```python
from build123d import *

# Parameters (mm, degrees)
BOSS_EXTRUDE1_DEPTH = 25.4
CUT_EXTRUDE1_REACH  = 3.587
SKETCH2_R           = 9.525
FILLET1_R           = 6.35
CUT_EXTRUDE2_REACH  = 33.75
SKETCH3_R           = 2.667


with BuildPart() as part:
    # Sketch1 → Boss-Extrude1 (new body)
    with BuildSketch(Plane(origin=(0, 0, 0), x_dir=(0, 0, -1), z_dir=(1, 0, 0))):
        Polygon((1.5875, 1.5875), (25.4, 1.5875), (25.4, 0), (0, 0), (0, 31.75), (1.5875, 31.75), align=None)
    extrude(amount=BOSS_EXTRUDE1_DEPTH)

    # Sketch2 → Cut-Extrude1 (cut, up to next)
    with BuildSketch(Plane(origin=(0, 0, -1.5875), x_dir=(-1, 0, 0), z_dir=(0, 0, -1)), mode=Mode.PRIVATE) as cut_extrude1_sk1:
        with Locations((-12.7, 18.830747356)):
            Circle(SKETCH2_R)
    cut_extrude1_tool1 = extrude(cut_extrude1_sk1.sketch, amount=-CUT_EXTRUDE1_REACH, mode=Mode.PRIVATE) & part.part
    add(cut_extrude1_tool1.solids().sort_by_distance((12.7, 18.830747, -1.5875))[0], mode=Mode.SUBTRACT)

    # Fillet1
    fillet1_edges = [part.edges().sort_by_distance(p)[0] for p in [
        (25.4, 31.75, -0.79375),
        (0, 31.75, -0.79375),
    ]]
    fillet(fillet1_edges, radius=FILLET1_R)

    # Sketch3 → Cut-Extrude2 (cut, up to next)
    with BuildSketch(Plane.XZ, mode=Mode.PRIVATE) as cut_extrude2_sk1:
        with Locations((17.653, -20.6375)):
            Circle(SKETCH3_R)
    cut_extrude2_tool1 = extrude(cut_extrude2_sk1.sketch, amount=-CUT_EXTRUDE2_REACH, mode=Mode.PRIVATE) & part.part
    add(cut_extrude2_tool1.solids().sort_by_distance((17.653, 0, -20.6375))[0], mode=Mode.SUBTRACT)
    # Sketch3 → Cut-Extrude2 (cut, up to next)
    with BuildSketch(Plane.XZ, mode=Mode.PRIVATE) as cut_extrude2_sk2:
        with Locations((10.287, -12.7)):
            Circle(SKETCH3_R)
    cut_extrude2_tool2 = extrude(cut_extrude2_sk2.sketch, amount=-CUT_EXTRUDE2_REACH, mode=Mode.PRIVATE) & part.part
    add(cut_extrude2_tool2.solids().sort_by_distance((10.287, 0, -12.7))[0], mode=Mode.SUBTRACT)


solid = part.part
```
Build history of the part. All positions in model axes, mm. A direction names the side the tool comes from. Round coordinates to 2 decimals unless told otherwise and drop trailing zeros. Write each loop counter-clockwise with the first axis right and the second up, starting at its lowest first coordinate (ties: lowest second). Pieces come first, ordered by that corner, then holes. Notation, with made-up numbers: (1, -15.75) -> (33, -15.75) arc R9 ccw to (33, 0.25) -> close; hole circle Ø8 at (-11.5, 67). An arc over 180 degrees is marked (long way). Put each result on its own line as item: value.
Item 1: Flat gauge pins, fed straight in: P1, Ø10, axis at x = 22.5, z = -20.5, coming from the +Y side; P2, Ø3, axis at x = 17.65, z = -20.64, coming from the -Y side; P3, Ø10, axis at x = 5.5, y = 14.5, coming from the -Z side. Where does each tip first touch, or does it go through?
Here are the results:
P1: stops at y = 1.59
P2: passes through
P3: stops at z = -1.59
Item 2: Slice it at C-C, the plane y = 14.5. Give the cut face in (x, z).
Here are the results:
outline: (0, -1.59) -> (4.22, -1.59) -> (4.22, 0) -> (0, 0) -> close; (21.18, -1.59) -> (25.4, -1.59) -> (25.4, 0) -> (21.18, 0) -> close
Item 3: Wall check: probe 1 along Y at (x, z) = (4.25, -8); probe 2 along Z at (x, y) = (7, 11); probe 3 along Y at (x, z) = (12.7, -1). Give the ranges that are in metal, low to high. Write a range as from..to.
Here are the results:
probe 1: y = 0..1.59
probe 2: z = -1.59..0
probe 3: y = 0..9.31, 28.36..31.75
Item 4: Slice it at D-D, the plane x = 21.75. Give the cut face in (y, z).
Here are the results:
outline: (0, -25.4) -> (1.59, -25.4) -> (1.59, -1.59) -> (15.86, -1.59) -> (15.86, 0) -> (0, 0) -> close; (21.8, -1.59) -> (31.15, -1.59) -> (31.15, 0) -> (21.8, 0) -> close
Item 5: Tool access for faces 1 (the face through (0, 1, -7)), 2 (the face through (18, 10, -1.588)): list every direction of +Z, -Z, +X, -X, +Y, -Y with a clear straight run to the whole face (end or side of a thin tool).
Here are the results:
face 1: +Z, -Z, -X, +Y, -Y
face 2: -Z, +X, -X, +Y
Item 6: Slice it at B-B, the plane x = 6.75. Give the cut face in (y, z), plus the area to 3 significant figures.
Here are the results:
outline: (0, -25.4) -> (1.59, -25.4) -> (1.59, -1.59) -> (11.39, -1.59) -> (11.39, 0) -> (0, 0) -> close; (26.27, -1.59) -> (31.75, -1.59) -> (31.75, 0) -> (26.27, 0) -> close
area: 64.6 mm^2
Item 7: Slice it at A-A, the plane z = -12.7. Give the cut face in (x, y), plus the area to 3 significant figures.
Here are the results:
outline: (0, 0) -> (7.62, 0) -> (7.62, 1.59) -> (0, 1.59) -> close; (12.95, 0) -> (25.4, 0) -> (25.4, 1.59) -> (12.95, 1.59) -> close
area: 31.9 mm^2
Item 8: Two-plate mould, pull along Y, no slides. Class faces 3 (the face through (13, 0, -10)), 4 (the face through (25.4, 1, -7)), 5 (the face through (14.76, 9.53, -0.8)), 6 (the face through (23.59, 29.84, -0.8)): pulls with the +Y half, pulls with the -Y half, needs draft (parallel to the pull), parting line crosses it, or undercut.
Here are the results:
face 3: pulls with the -Y half
face 4: needs draft
face 5: undercut
face 6: pulls with the +Y half
